Verification items for the finished model (mm, model axes). A direction names the side the tool comes from. Give positions to 0.01 mm unless a question says otherwise; leave off trailing zeros. Write each loop counter-clockwise with the first axis right and the second up, starting at its lowest first coordinate (ties: lowest second). Pieces come first, ordered by that corner, then holes. Notation, with made-up numbers: (48.5, 60) -> (72.5, 60) arc R10 cw to (72.5, 76) -> close; hole circle Ø4 at (19.25, -31). An arc over 180 degrees is marked (long way). Answer as CSV lines item,"result". Start each with the question number.
1) Mould release check, pull along Y, two halves, no side actions. Record for faces 1 (the flat face through (-20.25, -7, 10)), 2 (the flat face through (9, 24.165, 10)), 3 (the flat face through (24, 7.215, 10)): released by +Y, released by -Y, zero draft, split by the parting line, or undercut.
2) Sectioned sample at B-B on x = 9.45. Record the cut outline in (y, z) (3 decimals).
3) Gauge pin test, flat ends, axial feed: pin 1 Ø5 at (x, z) = (25.5, 10.5) entering from -Y (3 decimals); pin 2 Ø5 at (x, z) = (23, 3.5) entering from -Y (3 decimals); pin 3 Ø3 at (y, z) = (16, 10) entering from -X; pin 4 Ø8 at (x, z) = (-22.5, 11.5) entering from -Y (3 decimals). Record the tip position at first contact, or that the pin passes through.
4) Sectioned sample at D-D on z = 17.5. Record the cut outline in (x, y) (3 decimals).
5) Sectioned sample at A-A on z = 10.3. Record the cut outline in (x, y) (3 decimals), and give its area (3 significant figures).
6) Tool access check on faces 4 (the flat face through (25, -14, 7.23)), 5 (the flat face through (20.25, 15, 10)), 6 (the cylindrical face through (12.112, 22.188, 8.916)), 7 (the flat face through (-24, 7.215, 10)), 8 (the flat face through (-24, 10.465, 10)). Record the directions out of +Z, -Z, +X, -X, +Y, -Y that give a thin tool (end or side, any length) a straight path to the whole face; none if there is none.
7) Sectioned sample at C-C on y = 21.5. Record the cut outline in (x, z), and give its area (3 significant figures).
8) Material ranges on L1, parallel to Y at x = 22.5, z = 12.5 (3 decimals); L2, parallel to X at y = -12, z = 15.5; L3, parallel to Y at x = 1, z = 13.5 (3 decimals), recorded low to high.
```python
from build123d import *

# Parameters (mm, degrees)
SKETCH1_W           = 40.5
SKETCH1_H           = 40.53
BOSS_EXTRUDE1_DEPTH = 20.6
BOSS_EXTRUDE2_START = -9.8
SKETCH2_W           = 7.5
SKETCH2_H           = 20.6
BOSS_EXTRUDE2_DEPTH = 3.25
SKETCH3_R           = 3
BOSS_EXTRUDE3_DEPTH = 3.9
SKETCH4_W           = 6.14
SKETCH4_H           = 3.64
BOSS_EXTRUDE4_DEPTH = 9


with BuildPart() as part:
    # Sketch1 → Boss-Extrude1 (new body)
    with BuildSketch(Plane.XY):
        Rectangle(SKETCH1_W, SKETCH1_H)
    extrude(amount=BOSS_EXTRUDE1_DEPTH)

    # Sketch2 → Boss-Extrude2 (add)
    with BuildSketch(Plane(origin=(0, 20.265, 0), x_dir=(1, 0, 0), z_dir=(0, 1, 0)).offset(BOSS_EXTRUDE2_START)):
        with Locations((-24, -10.3)):
            Rectangle(SKETCH2_W, SKETCH2_H)
        with Locations((24, -10.3)):
            Rectangle(SKETCH2_W, SKETCH2_H)
    extrude(amount=-BOSS_EXTRUDE2_DEPTH)

    # Sketch3 → Boss-Extrude3 (add)
    with BuildSketch(Plane(origin=(0, 20.265, 0), x_dir=(1, 0, 0), z_dir=(0, 1, 0))):
        with Locations(Location((9.45, -10.3, 0), (0, 0, 90))):
            Circle(SKETCH3_R)
    extrude(amount=BOSS_EXTRUDE3_DEPTH)

    # Sketch4 → Boss-Extrude4 (add)
    with BuildSketch(Plane(origin=(20.25, 0, 0), x_dir=(0, 0, -1), z_dir=(1, 0, 0))):
        with Locations((-10.3, -14.165)):
            Rectangle(SKETCH4_W, SKETCH4_H)
    extrude(amount=BOSS_EXTRUDE4_DEPTH)


solid = part.part
```
Ans:
1,face 1,"zero draft"
1,face 2,"released by +Y"
1,face 3,"undercut"
2,outline,"(-20.265, 0) -> (20.265, 0) -> (20.265, 7.3) -> (24.165, 7.3) -> (24.165, 13.3) -> (20.265, 13.3) -> (20.265, 20.6) -> (-20.265, 20.6) -> close"
3,pin 1,"stops at y = -15.985"
3,pin 2,"stops at y = 7.215"
3,pin 3,"stops at x = -20.25"
3,pin 4,"stops at y = -20.265"
4,outline,"(-27.75, 7.215) -> (-20.25, 7.215) -> (-20.25, -20.265) -> (20.25, -20.265) -> (20.25, 7.215) -> (27.75, 7.215) -> (27.75, 10.465) -> (20.25, 10.465) -> (20.25, 20.265) -> (-20.25, 20.265) -> (-20.25, 10.465) -> (-27.75, 10.465) -> close"
5,outline,"(-27.75, 7.215) -> (-20.25, 7.215) -> (-20.25, -20.265) -> (20.25, -20.265) -> (20.25, -15.985) -> (29.25, -15.985) -> (29.25, -12.345) -> (20.25, -12.345) -> (20.25, 7.215) -> (27.75, 7.215) -> (27.75, 10.465) -> (20.25, 10.465) -> (20.25, 20.265) -> (12.45, 20.265) -> (12.45, 24.165) -> (6.45, 24.165) -> (6.45, 20.265) -> (-20.25, 20.265) -> (-20.25, 10.465) -> (-27.75, 10.465) -> close"
5,area,"1,750 mm²"
6,face 4,"-Z, +X, -Y"
6,face 5,"+Z, -Z, +X, +Y"
6,face 6,"+Y"
6,face 7,"+Z, -Z, -X, -Y"
6,face 8,"+Z, -Z, -X, +Y"
7,outline,"circle Ø6 at (9.45, 10.3)"
7,area,"28.3 mm²"
8,L1,"y = -15.985 to -12.345, 7.215 to 10.465"
8,L2,"x = -20.25 to 20.25"
8,L3,"y = -20.265 to 20.265"
